from build123d import *

# Parameters (mm, degrees)
F2_R     = 4.88099
F3_DEPTH = 5.6077
F4_DEPTH = 25.4
F1_R     = 6.18197
F5_DEPTH = 25.4


with BuildPart() as f3:
    # F2 (on face) → F3 (new body)
    with BuildSketch(Plane.XZ):
        Polygon((8.64374, 22.38507), (0, 22.38507), (-8.64374, 22.38507), (-8.64374, -23.271605), (-18.395651, -23.271605), (-18.395651, -37.234571), (0, -37.234571), (18.395651, -37.234571), (18.395651, -23.271605), (8.64374, -23.271605), align=None)
        with Locations((0, 11.968255)):
            Circle(F2_R, mode=Mode.SUBTRACT)
        with Locations((0, 11.968255)):
            Circle(F2_R)
    extrude(amount=F3_DEPTH)

    # F2 (on face) → F4 (cut)
    with BuildSketch(Plane.XZ):
        with Locations((0, 11.968255)):
            Circle(F2_R)
    extrude(amount=F4_DEPTH, mode=Mode.SUBTRACT)

    # F1 (on face) → F5 (cut)
    with BuildSketch(Plane.XZ):
        with Locations((0, -29.699003)):
            Circle(F1_R)
    extrude(amount=F5_DEPTH, mode=Mode.SUBTRACT)


solid = f3.part
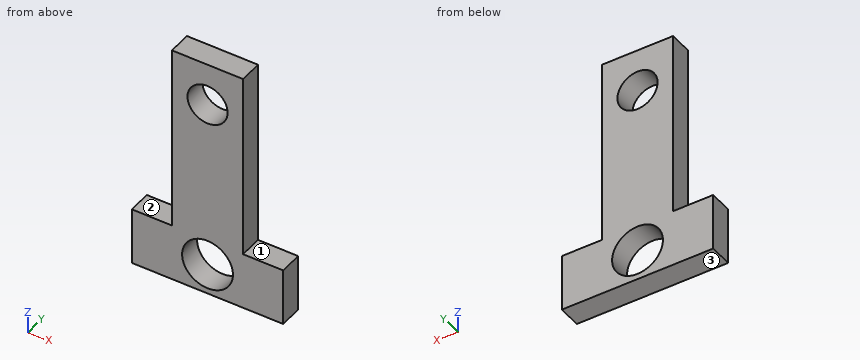
Here's how the part is built. I have some questions about the finished solid (model axes, mm). Face numbers are marked on the shaded views. A direction names the side the tool comes from. Coordinates: 2 decimals unless noted, no trailing zeros. Order: outer loops, then holes, each group sorted by start corner. A loop starts at its lowest first (then second) coordinate and runs counter-clockwise, first axis right, second up.
Item 1: If we section it at C-C on y = -4.05: List the corners of the cut face in (x, z) for me.
Result sheet:
outline: (-18.4, -37.23) - (18.4, -37.23) - (18.4, -23.27) - (8.64, -23.27) - (8.64, 22.39) - (-8.64, 22.39) - (-8.64, -23.27) - (-18.4, -23.27) - close; hole circle Ø12.36 at (0, -29.7); hole circle Ø9.76 at (0, 11.97)
Item 2: If we section it at A-A on x = -2: List the corners of the cut face in (y, z) for me.
Result sheet:
outline: (-5.61, -37.23) - (0, -37.23) - (0, -35.55) - (-5.61, -35.55) - close; (-5.61, -23.85) - (0, -23.85) - (0, 7.52) - (-5.61, 7.52) - close; (-5.61, 16.42) - (0, 16.42) - (0, 22.39) - (-5.61, 22.39) - close
Item 3: If we section it at B-B on z = -30.5: List the corners of the cut face in (x, y) for me, plus the area to 3 significant figures.
Result sheet:
outline: (-18.4, -5.61) - (-6.13, -5.61) - (-6.13, 0) - (-18.4, 0) - close; (6.13, -5.61) - (18.4, -5.61) - (18.4, 0) - (6.13, 0) - close
area: 138 mm2
Item 4: If we section it at D-D on x = -15: List the corners of the cut face in (y, z) for me, plus the area to 3 significant figures.
Result sheet:
outline: (-5.61, -37.23) - (0, -37.23) - (0, -23.27) - (-5.61, -23.27) - close
area: 78.3 mm2
Item 5: For P1, Ø3, axis at x = 12, y = -2, coming from the +Z side, with a flat end and sliding along its axis, tell me the tip position at first contact or that it passes through.
Result sheet:
P1: stops at z = -23.27
Item 6: I need wall thicknesses on line 1 (Z direction, x = 0, y = -2.8); line 2 (Z direction, x = -4, y = -3.2); line 3 (Z direction, x = 11, y = -3.6). Which ranges of each line are inside material? Lowest first, please.
Result sheet:
line 1: z = -37.23 to -35.88, -23.52 to 7.09, 16.85 to 22.39
line 2: z = -37.23 to -34.41, -24.99 to 9.17, 14.77 to 22.39
line 3: z = -37.23 to -23.27
Item 7: For the marked faces 1, 2 and 3, which set-ups out of +Z, -Z, +X, -X, +Y, -Y let a thin tool reach every point of the face, with its end or its side?
Result sheet:
face 1: +Z, +X, +Y, -Y
face 2: +Z, -X, +Y, -Y
face 3: -Z, +X, -X, +Y, -Y
